Input: part model. Units: mm. Frame: model coordinates. A direction names the side the tool comes from. Coordinates: 2 decimals unless noted, no trailing zeros. Write each loop counter-clockwise with the first axis right and the second up, starting at its lowest first coordinate (ties: lowest second). Pieces come first, ordered by that corner, then holes. Notation, with made-up numbers: M 81.25,-10.5 L 135.25,-10.5 A26 cw 135.25,18.5 Z; hole C 48,-10.5 d9. An arc over 180 degrees is marked long. Answer as a JSON object with one key per item and string values. Group by question number.
from build123d import *

# Parameters (mm, degrees)
BOSS_EXTRUDE1_DEPTH       = 5
M3X0_5_TAPPED_HOLE1_D     = 2.5
M3X0_5_TAPPED_HOLE1_DEPTH = 3
M3X0_5_TAPPED_HOLE1_TIP   = 0.751075774
BOSS_EXTRUDE2_DEPTH       = 5
CUT_EXTRUDE1_DEPTH        = 6
CUT_EXTRUDE2_DEPTH        = 6
BOSS_EXTRUDE3_DEPTH       = 5
BOSS_EXTRUDE4_DEPTH       = 5
SKETCH15_W                = 42.426406872
SKETCH15_H                = 0.46
BOSS_EXTRUDE6_DEPTH       = 5
SKETCH16_W                = 0.46
SKETCH16_H                = 42.886406871
BOSS_EXTRUDE7_DEPTH       = 5
M2X0_4_TAPPED_HOLE1_D     = 1.6
M2X0_4_TAPPED_HOLE1_DEPTH = 6
M2X0_4_TAPPED_HOLE1_TIP   = 0.480688495
SKETCH21_W                = 42.886406872
SKETCH21_H                = 1.7
CUT_EXTRUDE3_DEPTH        = 6
M3X0_5_TAPPED_HOLE3_D     = 2.5
M3X0_5_TAPPED_HOLE3_DEPTH = 6
M3X0_5_TAPPED_HOLE3_TIP   = 0.751075774


with BuildPart() as part:
    # Sketch2 → Boss-Extrude1 (new body)
    with BuildSketch(Plane.XY):
        Polygon((-19.445436483, 19.445436483), (26.516504294, -26.516504294), (-19.445436483, -26.516504294), align=None)
    extrude(amount=BOSS_EXTRUDE1_DEPTH)

    # M3x0.5 Tapped Hole1
    with Locations(Plane(origin=(0, 0, 0), x_dir=(0, 0, -1), z_dir=(0.707106781, 0.707106781, 0))):
        with Locations((-2.25, 19.75), (-2.25, -29.75)):
            Hole(M3X0_5_TAPPED_HOLE1_D / 2, depth=M3X0_5_TAPPED_HOLE1_DEPTH)
            with Locations((0, 0, -(M3X0_5_TAPPED_HOLE1_DEPTH + M3X0_5_TAPPED_HOLE1_TIP / 2))):  # 118° drill point
                Cone(0, M3X0_5_TAPPED_HOLE1_D / 2, M3X0_5_TAPPED_HOLE1_TIP, mode=Mode.SUBTRACT)

    # Sketch6 → Boss-Extrude2 (add, through all)
    with BuildSketch(Plane.XY.offset(5)):
        Polygon((-19.445436483, 19.445436483), (-15.909902577, 15.909902577), (-14.495689014, 17.324116139), (-18.03122292, 20.859650045), align=None)
        Polygon((26.516504294, -26.516504294), (22.980970389, -22.980970389), (24.395183951, -21.566756826), (27.930717857, -25.102290732), align=None)
    extrude(amount=-BOSS_EXTRUDE2_DEPTH)

    # Sketch7 → Cut-Extrude1 (cut, through all)
    with BuildSketch(Plane.XY.offset(5)):
        Polygon((-2.050609665, 2.050609665), (-5.586143571, -1.48492424), (13.081475452, -20.152543264), (16.617009358, -16.617009358), align=None)
    extrude(amount=-CUT_EXTRUDE1_DEPTH, mode=Mode.SUBTRACT)

    # Sketch9 → Cut-Extrude2 (cut, through all)
    with BuildSketch(Plane.XY.offset(5)):
        Polygon((-15.909902577, 15.909902577), (-19.445436483, 12.374368671), (-19.445436483, 19.445436483), (-18.03122292, 20.859650045), (-14.495689014, 17.324116139), align=None)
        Polygon((27.930717857, -25.102290732), (24.395183951, -21.566756826), (19.445436483, -26.516504294), (26.516504294, -26.516504294), align=None)
    extrude(amount=-CUT_EXTRUDE2_DEPTH, mode=Mode.SUBTRACT)

    # Sketch13 → Boss-Extrude3 (add, through all)
    with BuildSketch(Plane.XY.offset(5)):
        Polygon((22.980970389, -22.980970389), (19.445436483, -26.516504294), (22.980970389, -26.516504294), align=None)
    extrude(amount=-BOSS_EXTRUDE3_DEPTH)

    # Sketch14 → Boss-Extrude4 (add, through all)
    with BuildSketch(Plane.XY.offset(5)):
        Polygon((-19.445436483, 12.374368671), (-19.445436483, 15.909902577), (-15.909902577, 15.909902577), align=None)
    extrude(amount=-BOSS_EXTRUDE4_DEPTH)

    # Sketch15 → Boss-Extrude6 (add, through all)
    with BuildSketch(Plane(origin=(0, 0, 0), x_dir=(-1, 0, 0), z_dir=(0, 0, -1))):
        with Locations((-1.767766953, -26.746504294)):
            Rectangle(SKETCH15_W, SKETCH15_H)
    extrude(amount=-BOSS_EXTRUDE6_DEPTH)

    # Sketch16 → Boss-Extrude7 (add, through all)
    with BuildSketch(Plane(origin=(0, 0, 0), x_dir=(-1, 0, 0), z_dir=(0, 0, -1))):
        with Locations((19.675436483, -5.533300859)):
            Rectangle(SKETCH16_W, SKETCH16_H)
    extrude(amount=-BOSS_EXTRUDE7_DEPTH)

    # M2x0.4 Tapped Hole1
    with Locations(Plane(origin=(0, 0, 0), x_dir=(-1, 0, 0), z_dir=(0, 0, -1))):
        with Locations((17.70619852, -11.976504294), (17.70619852, -21.976504294)):
            Hole(M2X0_4_TAPPED_HOLE1_D / 2, depth=M2X0_4_TAPPED_HOLE1_DEPTH)
            with Locations((0, 0, -(M2X0_4_TAPPED_HOLE1_DEPTH + M2X0_4_TAPPED_HOLE1_TIP / 2))):  # 118° drill point
                Cone(0, M2X0_4_TAPPED_HOLE1_D / 2, M2X0_4_TAPPED_HOLE1_TIP, mode=Mode.SUBTRACT)

    # Sketch21 → Cut-Extrude3 (cut, through all)
    with BuildSketch(Plane.XY.offset(5)):
        with Locations((1.537766953, -26.126504294)):
            Rectangle(SKETCH21_W, SKETCH21_H)
    extrude(amount=-CUT_EXTRUDE3_DEPTH, mode=Mode.SUBTRACT)

    # M3x0.5 Tapped Hole3
    with Locations(Plane(origin=(0, -25.276504294, 0), x_dir=(-1, 0, 0), z_dir=(0, -1, 0))):
        with Locations((7.905436483, -2.5), (-7.094563517, -2.5)):
            Hole(M3X0_5_TAPPED_HOLE3_D / 2, depth=M3X0_5_TAPPED_HOLE3_DEPTH)
            with Locations((0, 0, -(M3X0_5_TAPPED_HOLE3_DEPTH + M3X0_5_TAPPED_HOLE3_TIP / 2))):  # 118° drill point
                Cone(0, M3X0_5_TAPPED_HOLE3_D / 2, M3X0_5_TAPPED_HOLE3_TIP, mode=Mode.SUBTRACT)


solid = part.part
Q1. Draft query along X for faces 1 (the conical face through (6.888, -18.656, 2.435)), 2 (the flat face through (20, -20, 2)), 3 (the flat face through (-8, -9, 0)). Return one class per face: released by +X, released by -X, zero draft, split by the parting line, or undercut.
Q2. Section C-C, the plane y = -15.5. Return the cut outline in (x, z).
Q3. Section D-D, the plane x = 12. Return the cut outline in (y, z), and give its area (3 significant figures).
Q4. Access query for faces 4 (the cylindrical face through (8.287, -22.235, 2.125)), 5 (the conical face through (-16.376, 11.255, 2.297)), 6 (the flat face through (3.62, -10.69, 2.54)), 7 (the flat face through (14.824, -18.41, 2.535)), 8 (the flat face through (-3.8, 0.3, 2.5)). Directions: +Z, -Z, +X, -X, +Y, -Y. A direction counts if a zero-diameter tool reaches every point of the face in a straight line with its end or side. Return the directions, or none.
Q5. Line query: line 1 (Y direction, x = -17, z = 4.2); line 2 (X direction, y = 12, z = 1.95); line 3 (X direction, y = -4, z = 0.65). Output: solid intervals per line, ascending. Write a range as from..to.
Q6. Pin query (flat end, axial travel): pin 1 Ø1.4 at (x, y) = (-17.71, -11.98) entering from -Z; pin 2 Ø1.5 at (x, z) = (7.09, 2.5) entering from -Y. Return the tip coordinate at first contact, or that it passes through.
Q7. Section A-A, the plane x = -4.5. Return the cut outline in (y, z).
Q8. Section B-B, the plane z = 4.3. Return the cut outline in (x, y), and give its area (3 significant figures).
Filled in:
{
 "1": {"face 1": "undercut", "face 2": "released by +X", "face 3": "zero draft"},
 "2": {"outline": "M -19.91,0 L 8.43,0 L 8.43,5 L -19.91,5 Z"},
 "3": {"outline": "M -25.28,0 L -19.07,0 L -19.07,5 L -25.28,5 Z", "area": "31.0 mm^2"},
 "4": {"face 4": "-Y", "face 5": "none", "face 6": "+Z, -Z", "face 7": "+Z, -Z, +Y", "face 8": "+Z, -Z, +X"},
 "5": {"line 1": "-25.28..-22.35, -21.6..-12.35, -11.6..15.91", "line 2": "-19.91..-16.75, -14.21..-12", "line 3": "-19.91..-3.07"},
 "6": {"pin 1": "through", "pin 2": "y = -18.98"},
 "7": {"outline": "M -25.28,0 L -2.57,0 L -2.57,5 L -25.28,5 Z; M -0.4,0 L 4.5,0 L 4.5,5 L -0.4,5 Z"},
 "8": {"outline": "M -19.91,-25.28 L 22.98,-25.28 L 22.98,-22.98 L 16.62,-16.62 L 13.08,-20.15 L -5.59,-1.48 L -2.05,2.05 L -15.91,15.91 L -19.91,15.91 Z; hole C -17.71,-21.98 d1.6; hole C -17.71,-11.98 d1.6", "area": "874 mm^2"}
}
